from build123d import *

# Parameters (mm, degrees)
F1_DEPTH = 19.812
F2_SIZE  = 5.08
F3_SIZE  = 5.08


with BuildPart() as f1:
    # F0 (on Top) → F1 (new body)
    with BuildSketch(Plane.XY):
        Polygon((-58.608726, -45.600105), (-58.608726, -49.796436), (-16.645437, -50.076187), (-16.645437, -42.522795), (-23.311197, -42.522795), (-23.311197, -25.737481), (-23.311197, -11.458973), (-29.514179, -7.553392), (-24.758339, 0), (43.50194, 6.43437), (43.50194, 15.666293), (50.775576, 15.666293), (50.775576, 23.49944), (41.263901, 23.49944), (38.186591, 28.535035), (-52.174356, 28.535035), (-55.531416, 23.49944), (-67.840651, 18.743601), (-67.840651, 11.469965), (-62.805057, 15.666293), (-55.531416, 15.666293), (-55.531416, -45.600105), align=None)
    extrude(amount=F1_DEPTH)

    # F2
    f2_edges = [f1.edges().sort_by_distance(p)[0] for p in [
        (-6.993882, 28.535035, 19.812),
        (9.3718, 3.217185, 19.812),
        (-55.531416, -14.966906, 19.812),
        (-23.311197, -26.990884, 19.812),
        (-26.412688, -9.506182, 19.812),
        (-27.136259, -3.776696, 19.812),
    ]]
    chamfer(f2_edges, length=F2_SIZE)

    # F3
    f3_edges = [f1.edges().sort_by_distance(p)[0] for p in [
        (-55.531416, -14.966906, 0),
        (-6.993882, 28.535035, 0),
        (9.3718, 3.217185, 0),
        (-23.311197, -26.990884, 0),
        (-26.412688, -9.506182, 0),
        (-27.136259, -3.776696, 0),
    ]]
    chamfer(f3_edges, length=F3_SIZE)


solid = f1.part
Geometry check sheet. Reference: the model listing, model coordinates, mm. A direction names the side the tool comes from. Give positions to 0.01 mm unless a question says otherwise; leave off trailing zeros. Loops run counter-clockwise (first coordinate to the right, second up) from the corner with the lowest first, then second, coordinate; pieces in that order, holes last.
(1) Section check C-C on x = 8.5. Record the cut outline in (y, z) (3 decimals), then the cut area to 3 significant figures.
From the geometry:
outline: (3.135, 5.08) - (8.238, 0) - (23.455, 0) - (28.535, 5.08) - (28.535, 14.732) - (23.455, 19.812) - (8.238, 19.812) - (3.135, 14.732) - close
area: 451 mm2
(2) Section check B-B on y = -25. Record the cut outline in (x, z), then the cut area to 3 significant figures.
From the geometry:
outline: (-55.53, 5.08) - (-50.45, 0) - (-28.39, 0) - (-23.31, 5.08) - (-23.31, 14.73) - (-28.39, 19.81) - (-50.45, 19.81) - (-55.53, 14.73) - close
area: 587 mm2
(3) Section check A-A on z = 13.25. Record the cut outline in (x, y), then the cut area to 3 significant figures.
From the geometry:
outline: (-67.84, 11.47) - (-62.81, 15.67) - (-55.53, 15.67) - (-55.53, -45.6) - (-58.61, -45.6) - (-58.61, -49.8) - (-16.65, -50.08) - (-16.65, -42.52) - (-23.31, -42.52) - (-23.31, -11.46) - (-29.51, -7.55) - (-24.76, 0) - (43.5, 6.43) - (43.5, 15.67) - (50.78, 15.67) - (50.78, 23.5) - (41.26, 23.5) - (38.19, 28.54) - (-52.17, 28.54) - (-55.53, 23.5) - (-67.84, 18.74) - close
area: 4,340 mm2
(4) Section check D-D on z = 2. Record the cut outline in (x, y).
From the geometry:
outline: (-67.84, 11.47) - (-62.81, 15.67) - (-52.45, 15.67) - (-52.45, -45.6) - (-58.61, -45.6) - (-58.61, -49.8) - (-16.65, -50.08) - (-16.65, -42.52) - (-26.39, -42.52) - (-26.39, -13.16) - (-33.76, -8.52) - (-26.56, 2.92) - (43.5, 9.53) - (43.5, 15.67) - (50.78, 15.67) - (50.78, 23.5) - (41.26, 23.5) - (40.07, 25.46) - (-54.23, 25.46) - (-55.53, 23.5) - (-67.84, 18.74) - close
(5) Release check for a two-part mould opening along Y. For faces 4 (the flat face through (46, 23.499, 10)), 5 (the flat face through (-52.956, -14.538, 17.308)), 6 (the flat face through (-58, 15.666, 10)), 7 (the flat face through (-36, -5, 19.812)) record: released by +Y, released by -Y, zero draft, split by the parting line, or undercut.
From the geometry:
face 4: released by +Y
face 5: undercut
face 6: undercut
face 7: zero draft
(6) Depth check by flat-ended pin: pin 1 Ø10 at (x, z) = (35.5, 9) entering from -Y; pin 2 Ø2 at (y, z) = (-48, 10) entering from -X; pin 3 Ø3 at (y, z) = (11.5, 11) entering from +X. Enter the tip coordinate at first touch or a pass-through.
From the geometry:
pin 1: stops at y = 5.21
pin 2: stops at x = -58.61
pin 3: stops at x = 43.5
(7) Set-up check for faces 1 (the flat face through (-30.064, -3.594, 2.504)), 2 (the flat face through (-56, -45.6, 10)), 3 (the flat face through (47, 15.666, 10)): record each of +Z, -Z, +X, -X, +Y, -Y from which the full face is reachable in a straight line by a thin tool's end or side.
From the geometry:
face 1: -Z, +X
face 2: -X
face 3: +Z, -Z, +X, -Y
(8) Thickness scan on L1, parallel to X at y = -44, z = 14.5; L2, parallel to Y at x = -23, z = 14.25; L3, parallel to X at y = -42, z = 12. Record the ranges inside material, lowest first.
From the geometry:
L1: x = -55.53 to -16.65
L2: y = -50.03 to -42.52, 0.17 to 28.54
L3: x = -55.53 to -23.31
